from build123d import *

# Parameters (mm, degrees)
F1_DEPTH = 25.7
F2_W     = 20.5
F2_H     = 20.5
F3_DEPTH = 20
F4_W     = 20.5
F4_H     = 20.5
F5_DEPTH = 20


with BuildPart() as f1:
    # F0 (on Front) → F1 (new body)
    with BuildSketch(Plane.XZ):
        with BuildLine():
            Line((0.6698729811, -1.1602540378), (10.3245955671, -17.8827240898))
            Line((10.3245955671, -17.8827240898), (32.5814484444, -5.0327240898))
            Line((32.5814484444, -5.0327240898), (19.4835787356, 17.6534517167))
            ThreePointArc((19.4835787356, 17.6534517167), (18.6889856226, 18.6889856226), (17.6534517167, 19.4835787356))
            Line((17.6534517167, 19.4835787356), (-5.0327240898, 32.5814484444))
            Line((-5.0327240898, 32.5814484444), (-17.8827240898, 10.3245955671))
            Line((-17.8827240898, 10.3245955671), (-1.1602540378, 0.6698729811))
            ThreePointArc((-1.1602540378, 0.6698729811), (-0.1247201319, -0.1247201319), (0.6698729811, -1.1602540378))
        make_face()
    extrude(amount=F1_DEPTH)

    # F2 (on face) → F3 (cut)
    with BuildSketch(Plane(origin=(-17.8827240898, 0, 10.3245955671), x_dir=(0, -1, 0), z_dir=(-0.8660254038, 0, 0.5))):
        with Locations((12.85, 12.85)):
            Rectangle(F2_W, F2_H)
    extrude(amount=-F3_DEPTH, mode=Mode.SUBTRACT)

    # F4 (on face) → F5 (cut)
    with BuildSketch(Plane(origin=(10.3245955671, 0, -17.8827240898), x_dir=(0.8660254038, 0, 0.5), z_dir=(0.5, 0, -0.8660254038))):
        with Locations((12.85, 12.85)):
            Rectangle(F4_W, F4_H)
    extrude(amount=-F5_DEPTH, mode=Mode.SUBTRACT)


solid = f1.part
Model file for the job. Use its own axes, mm. A direction names the side the tool comes from. Give positions to 0.01 mm unless a question says otherwise; leave off trailing zeros. Order: outer loops, then holes, each group sorted by start corner. A loop starts at its lowest first (then second) coordinate and runs counter-clockwise, first axis right, second up. Notation, with made-up numbers: M -8,24.5 L 12,24.5 A22 ccw 12,30.5 Z; hole C 11,25.5 d11. An arc over 180 degrees is marked long. Put each result on its own line as item: value. Start each with the question number.
(1) Band-saw the part on D-D on x = -9.5. Give the cut face in (y, z), then the cut area to 3 significant figures.
(2) Tool access for faces 5 (the face through (7.646, -12.706, -8.044)), 6 (the face through (2.206, -12.706, 25.4)), 7 (the face through (25.4, -12.706, 2.206)): list every direction of +Z, -Z, +X, -X, +Y, -Y with a clear straight run to the whole face (end or side of a thin tool).
(3) Band-saw the part on B-B on z = 5. Give the cut face in (x, y).
(4) Drill centre lines: L1, parallel to Y at x = -9, z = 13; L2, parallel to X at y = -7.25, z = 10; L3, parallel to X at y = -21.5, z = -5. Where is each one in solid material? Low to high. Write a range as [from, to].
(5) Pull direction Y, two halves, no side cores. Call faces 1 (the face through (21.297, -1.248, -11.548)), 2 (the face through (7, -25.7, 8)), 3 (the face through (-8.044, -12.706, 7.646)), 4 (the face through (-3, -23.1, 16)): released by +Y, released by -Y, zero draft, split by the parting line, or undercut.
(6) Pin check, flat tips, straight feed: pin 1 Ø1.5 at (y, z) = (-15.5, 5) entering from -X; pin 2 Ø12 at (x, y) = (22.5, -10) entering from -Z; pin 3 Ø1.5 at (y, z) = (-3.5, 4.5) entering from -X. Stop position of each tip, or through.
(7) Band-saw the part on C-C on y = -8.5. Give the cut face in (x, z).
(8) Band-saw the part on A-A on x = 6. Give the cut face in (y, z).
Results below:
1. outline: M -25.7,5.48 L 0,5.48 L 0,24.84 L -2.6,24.84 L -2.6,8.49 L -23.1,8.49 L -23.1,24.84 L -25.7,24.84 Z
1. area: 162 mm2
2. face 5: none
2. face 6: -X
2. face 7: -Z
3. outline: M -8.66,-25.7 L 26.79,-25.7 L 26.79,0 L -8.66,0 Z; hole M -3.46,-23.1 L 2.14,-23.1 L 2.14,-2.6 L -3.46,-2.6 Z; hole M 9.96,-23.1 L 23.79,-23.1 L 23.79,-2.6 L 9.96,-2.6 Z
4. L1: y = [-25.7, -23.1], [-2.6, 0]
4. L2: x = [-17.32, -12.12], [5.02, 18.62], [20.9, 23.9]
4. L3: x = [2.89, 5.89], [29.56, 32.56]
5. face 1: zero draft
5. face 2: released by -Y
5. face 3: undercut
5. face 4: undercut
6. pin 1: stops at x = -9.96
6. pin 2: stops at z = -3.16
6. pin 3: stops at x = -9.09
7. outline: M -17.88,10.32 L -1.16,0.67 A5 cw 0.67,-1.16 L 10.32,-17.88 L 12.58,-16.58 L 2.58,0.74 L 20.33,10.99 L 30.33,-6.33 L 32.58,-5.03 L 19.48,17.65 A5 ccw 17.65,19.48 L -5.03,32.58 L -6.33,30.33 L 10.99,20.33 L 0.74,2.58 L -16.58,12.58 Z
8. outline: M -25.7,-10.39 L 0,-10.39 L 0,26.21 L -25.7,26.21 Z; hole M -23.1,-5.19 L -2.6,-5.19 L -2.6,2.71 L -23.1,2.71 Z; hole M -23.1,11.69 L -2.6,11.69 L -2.6,23.21 L -23.1,23.21 Z
